Build history of the part. All positions in model axes, mm. A direction names the side the tool comes from. Give positions to 0.01 mm unless a question says otherwise; leave off trailing zeros. Write each loop counter-clockwise with the first axis right and the second up, starting at its lowest first coordinate (ties: lowest second). Pieces come first, ordered by that corner, then holes. Notation, with made-up numbers: (-15.75, 1) - (23.25, 1) arc R10 ccw to (23.25, 8) - close; hole circle Ø6 at (41.5, 52). An arc over 180 degrees is marked (long way). Use one line per item in the form item = value. Start each with the question number.
from build123d import *

# Parameters (mm, degrees)
SKETCH1_W           = 45
SKETCH1_H           = 58
BOSS_EXTRUDE1_DEPTH = 8
FILLET1_R           = 7.5
SHELL1_START        = -28
SHELL1_DEPTH        = 56
SKETCH2_W           = 18
SKETCH2_H           = 15
SKETCH2_W_2         = 3
CUT_EXTRUDE1_DEPTH  = 55.129474411
BOSS_EXTRUDE2_DEPTH = 10


# Read off the part's stored shape, not the designer's step: Shell1
with BuildPart() as part:
    # Sketch1 → Boss-Extrude1 (new, symmetric)
    with BuildSketch(Plane(origin=(0, 0, 0), x_dir=(1, 0, 0), z_dir=(0, 1, 0))):
        Rectangle(SKETCH1_W, SKETCH1_H)
    extrude(amount=BOSS_EXTRUDE1_DEPTH, both=True)

    # Fillet1
    fillet1_edges = [part.edges().sort_by_distance(p)[0] for p in [
        (22.5, 8, 0),
        (-22.5, 8, 0),
    ]]
    fillet(fillet1_edges, radius=FILLET1_R)

    # Shell1 outline → Shell1 (cut)
    with BuildSketch(Plane.XY.offset(SHELL1_START)):
        with BuildLine():
            ThreePointArc((21.5, 0.5), (19.596194078, 5.096194078), (15, 7))
            Line((15, 7), (15, 8))
            Line((15, 8), (-15, 8))
            Line((-15, 8), (-15, 7))
            ThreePointArc((-15, 7), (-19.596194078, 5.096194078), (-21.5, 0.5))
            Line((-21.5, 0.5), (-21.5, -7))
            Line((-21.5, -7), (21.5, -7))
            Line((21.5, -7), (21.5, 0.5))
        make_face()
    extrude(amount=SHELL1_DEPTH, mode=Mode.SUBTRACT)

    # Sketch2 → Cut-Extrude1 (cut, through all)
    with BuildSketch(Plane(origin=(22.5, 0, 0), x_dir=(0, 0, -1), z_dir=(1, 0, 0))):
        with Locations((0, 5.7)):
            Rectangle(SKETCH2_W, SKETCH2_H)
        with Locations((-26.5, 5.7)):
            Rectangle(SKETCH2_W_2, SKETCH2_H)
        with Locations((26.5, 5.7)):
            Rectangle(SKETCH2_W_2, SKETCH2_H)
    extrude(amount=-CUT_EXTRUDE1_DEPTH, mode=Mode.SUBTRACT)

    # Sketch3 → Boss-Extrude2 (add)
    with BuildSketch(Plane(origin=(0, 0, -29), x_dir=(-1, 0, 0), z_dir=(0, 0, -1))):
        with BuildLine():
            ThreePointArc((18.940983006, -7), (20.25, -6.5), (18.940983006, -6))
            ThreePointArc((18.940983006, -6), (17.631966011, -6.5), (18.940983006, -7))
        make_face()
    extrude(amount=BOSS_EXTRUDE2_DEPTH)


solid = part.part
(1) Cut at D-D, the plane z = -31.5. Give the cut face in (x, y).
(2) Two-plate mould, pull along Z, no slides. Class faces 4 (the cylindrical face through (20.245, 5.861, 16.888)), 5 (the flat face through (-18.9, -6.5, -39)), 6 (the cylindrical face through (-19.545, 5.146, 16.888)): +Z half, -Z half, draft (parallel to the pull), parting line (faces both ways), or undercut.
(3) Which spindle directions (+Z, -Z, +X, -X, +Y, -Y) get a long thin tool onto all of the face, cutting with end or side? Do faces 1 (the flat face through (-20, 5, 9)), 2 (the flat face through (0, 0, 28)), 3 (the flat face through (21.5, -4, 0)). Say none if no direction does.
(4) Wall check: line 1 (Z direction, x = 13.5, y = 6.5); line 2 (X direction, y = -3, z = -5); line 3 (Y direction, x = 2.5, z = -0.5). Give the ranges that are in metal, low to high. Write a range as from..to.
(5) Pin check, flat tips, straight feed: pin 1 Ø7.5 at (x, y) = (-1, -2) entering from -Z; pin 2 Ø0.5 at (y, z) = (7.5, 15.5) entering from +X. Stop position of each tip, or through.
(6) Cut at A-A, the plane z = 18.5. Give the cut face in (x, y).
(7) Cut at C-C, the plane x = 16. Give the cut face in (y, z), then the cut area to 3 significant figures.
(8) Cut at B-B, the plane x = -13. Give the cut face in (y, z), then the cut area to 3 significant figures.
Solution:
q1.outline = (-18.94, -7) arc R0.75 ccw (long way) to (-18.94, -6) arc R0.75 ccw (long way) to start
q2.face_4 = draft
q2.face_5 = -Z half
q2.face_6 = undercut
q3.face_1 = +X, -X, +Y
q3.face_2 = +Y
q3.face_3 = none
q4.line_1 = -29..-28, 28..29
q4.line_2 = -22.5..-21.5, 21.5..22.5
q4.line_3 = -8..-7
q5.pin_1 = -29
q5.pin_2 = 18.27
q6.outline = (-22.5, -8) - (22.5, -8) - (22.5, 0.5) arc R7.5 ccw to (15, 8) - (15, 7) arc R6.5 cw to (21.5, 0.5) - (21.5, -7) - (-21.5, -7) - (-21.5, 0.5) arc R6.5 cw to (-15, 7) - (-15, 8) arc R7.5 ccw to (-22.5, 0.5) - close
q7.outline = (-8, -29) - (7.93, -29) - (7.93, -28) - (-7, -28) - (-7, 28) - (7.93, 28) - (7.93, 29) - (-8, 29) - close; (6.92, -25) - (7.93, -25) - (7.93, -9) - (6.92, -9) - close; (6.92, 9) - (7.93, 9) - (7.93, 25) - (6.92, 25) - close
q7.area = 120 mm2
q8.outline = (-8, -29) - (8, -29) - (8, -28) - (-7, -28) - (-7, 28) - (8, 28) - (8, 29) - (-8, 29) - close
q8.area = 88.0 mm2
